from build123d import *

# Parameters (mm, degrees)
SKETCH1_W                           = 42
SKETCH1_H                           = 42
BOSS_EXTRUDE1_DEPTH                 = 33
SKETCH2_R                           = 11
BOSS_EXTRUDE2_DEPTH                 = 2
SKETCH3_R                           = 2
BOSS_EXTRUDE3_DEPTH                 = 22
SKETCH4_W                           = 15
SKETCH4_H                           = 10
BOSS_EXTRUDE4_DEPTH                 = 7
F_2_0MM_CLEARANCE_DOWEL_HOLE1_D     = 2
F_2_0MM_CLEARANCE_DOWEL_HOLE1_DEPTH = 8
F_2_0MM_CLEARANCE_DOWEL_HOLE1_TIP   = 0.600860619
CHAMFER1_SIZE                       = 4


with BuildPart() as part:
    # Sketch1 → Boss-Extrude1 (new body)
    with BuildSketch(Plane(origin=(0, 0, 0), x_dir=(1, 0, 0), z_dir=(0, 1, 0))):
        with Locations((21, -21)):
            Rectangle(SKETCH1_W, SKETCH1_H)
    extrude(amount=BOSS_EXTRUDE1_DEPTH)

    # Sketch2 → Boss-Extrude2 (add)
    with BuildSketch(Plane(origin=(0, 33, 0), x_dir=(1, 0, 0), z_dir=(0, 1, 0))):
        with Locations(Location((21, -21, 0), (0, 0, 270))):
            Circle(SKETCH2_R)
    extrude(amount=BOSS_EXTRUDE2_DEPTH)

    # Sketch3 → Boss-Extrude3 (add)
    with BuildSketch(Plane(origin=(0, 35, 0), x_dir=(1, 0, 0), z_dir=(0, 1, 0))):
        with Locations(Location((21, -21, 0), (0, 0, 270))):
            Circle(SKETCH3_R)
    extrude(amount=BOSS_EXTRUDE3_DEPTH)

    # Sketch4 → Boss-Extrude4 (add)
    with BuildSketch(Plane.XY.offset(42)):
        with Locations((21, 5)):
            Rectangle(SKETCH4_W, SKETCH4_H)
    extrude(amount=BOSS_EXTRUDE4_DEPTH)

    # Ø2.0mm Clearance Dowel Hole1
    with Locations(Plane(origin=(37, 33, 5), x_dir=(0, 0, 1), z_dir=(0, 1, 0))):
        with Locations((0, 0), (32, 0), (32, -32), (0, -32)):
            Hole(F_2_0MM_CLEARANCE_DOWEL_HOLE1_D / 2, depth=F_2_0MM_CLEARANCE_DOWEL_HOLE1_DEPTH)
            with Locations((0, 0, -(F_2_0MM_CLEARANCE_DOWEL_HOLE1_DEPTH + F_2_0MM_CLEARANCE_DOWEL_HOLE1_TIP / 2))):  # 118° drill point
                Cone(0, F_2_0MM_CLEARANCE_DOWEL_HOLE1_D / 2, F_2_0MM_CLEARANCE_DOWEL_HOLE1_TIP, mode=Mode.SUBTRACT)

    # Chamfer1
    chamfer1_edges = [part.edges().sort_by_distance(p)[0] for p in [
        (0, 16.5, 0),
        (42, 16.5, 0),
        (42, 16.5, 42),
        (0, 16.5, 42),
    ]]
    chamfer(chamfer1_edges, length=CHAMFER1_SIZE)


solid = part.part
Verification items for the finished model (mm, model axes). A direction names the side the tool comes from. Coordinates: 2 decimals unless noted, no trailing zeros. Write each loop counter-clockwise with the first axis right and the second up, starting at its lowest first coordinate (ties: lowest second). Pieces come first, ordered by that corner, then holes. Notation, with made-up numbers: (36.5, 73) - (77.5, 73) arc R28 cw to (77.5, 109) - close; hole circle Ø1 at (46.5, 26.25). An arc over 180 degrees is marked (long way). Answer as a JSON object with one key per item and string values.
(1) Thickness scan on line 1 along Z through (x, y) = (5, 26.5); line 2 along Y through (x, z) = (13, 29.5). Record the ranges inside material, lowest first.
Report:
{"line 1": "0 to 4, 6 to 36, 38 to 42", "line 2": "0 to 33"}
(2) Cross-section at C-C on z = 46.5. Record the cut outline in (x, y).
Report:
{"outline": "(13.5, 0) - (28.5, 0) - (28.5, 10) - (13.5, 10) - close"}
(3) Tool access check on faces 1 (the flat face through (21, 10, 45)), 2 (the flat face through (21, 5, 49)), 3 (the flat face through (28.5, 5, 45)), 4 (the flat face through (21, 16, 0)), 5 (the cylindrical face through (37.84, 28.94, 36.46)). Record the directions out of +Z, -Z, +X, -X, +Y, -Y that give a thin tool (end or side, any length) a straight path to the whole face; none if there is none.
Report:
{"face 1": "+Z, +X, -X, +Y", "face 2": "+Z, +X, -X, +Y, -Y", "face 3": "+Z, +X, +Y, -Y", "face 4": "-Z, +X, -X, +Y, -Y", "face 5": "+Y"}
(4) Cross-section at D-D on x = 26. Record the cut outline in (y, z).
Report:
{"outline": "(0, 0) - (33, 0) - (33, 11.2) - (35, 11.2) - (35, 30.8) - (33, 30.8) - (33, 42) - (10, 42) - (10, 49) - (0, 49) - close"}
(5) Cross-section at A-A on y = 5.5. Record the cut outline in (x, z).
Report:
{"outline": "(0, 4) - (4, 0) - (38, 0) - (42, 4) - (42, 38) - (38, 42) - (28.5, 42) - (28.5, 49) - (13.5, 49) - (13.5, 42) - (4, 42) - (0, 38) - close"}
(6) Cross-section at B-B on x = 21. Record the cut outline in (y, z).
Report:
{"outline": "(0, 0) - (33, 0) - (33, 10) - (35, 10) - (35, 19) - (57, 19) - (57, 23) - (35, 23) - (35, 32) - (33, 32) - (33, 42) - (10, 42) - (10, 49) - (0, 49) - close"}
(7) Gauge pin test, flat ends, axial feed: pin 1 Ø5.5 at (x, z) = (22.5, 45) entering from +Y; pin 2 Ø1.6 at (x, z) = (5, 5) entering from +Y; pin 3 Ø6 at (x, y) = (7, 20.5) entering from +Z. Record the tip position at first contact, or that the pin passes through.
Report:
{"pin 1": "y = 10", "pin 2": "y = 24.88", "pin 3": "z = 42"}
(8) Mould release check, pull along X, two halves, no side actions. Record for faces 6 (the conical face through (37.01, 24.5, 36.83)), 7 (the flat face through (2, 16, 40)), 8 (the flat face through (18.7, 35, 20.8)): pulls with the +X half, pulls with the -X half, needs draft (parallel to the pull), parting line crosses it, or undercut.
Report:
{"face 6": "undercut", "face 7": "pulls with the -X half", "face 8": "needs draft"}
